from build123d import *

# Parameters (mm, degrees)
PAD_DEPTH = 8


with BuildPart() as part:
    # Sketch → Pad (new body)
    with BuildSketch(Plane.XY):
        with BuildLine():
            ThreePointArc((-29.53026, 52.229912), (0, -60), (29.53026, 52.229912))
            Line((29.53026, 122.229912), (29.53026, 52.229912))
            Line((23.53026, 122.229912), (29.53026, 122.229912))
            Line((23.53026, 122.229912), (23.53026, 82.229912))
            Line((23.53026, 82.229912), (-29.53026, 52.229912))
        make_face()
    extrude(amount=PAD_DEPTH)


solid = part.part
Here's how the part is built. I have some questions about the finished solid (model axes, mm). A direction names the side the tool comes from. Give positions to 0.01 mm unless a question says otherwise; leave off trailing zeros. Order: outer loops, then holes, each group sorted by start corner. A loop starts at its lowest first (then second) coordinate and runs counter-clockwise, first axis right, second up. Notation, with made-up numbers: M -27.75,75.5 L -1.75,75.5 A29 ccw -1.75,108.5 Z; hole C 71.5,25.25 d5. An arc over 180 degrees is marked long. Answer as a JSON object with one key per item and string values. Group by question number.
1) Please list where these lines run through material, in increasing order: L1, parallel to X at y = 84.5, z = 5.5; L2, parallel to Y at x = 12.5, z = 2; L3, parallel to Y at x = -46, z = 5.5. Write a range as [from, to].
2) Suppose I cut it at B-B, the plane x = 44.5. Write out the boundary of the cut face in (y, z), plus the area to 3 significant figures.
3) Suppose I cut it at A-A, the plane y = 93. Write out the boundary of the cut face in (x, z), plus the area to 3 significant figures.
4) On a 3-axis mill with a long thin cutter (end or side, diameter ignored), from which of +Z, -Z, +X, -X, +Y, -Y can I reach the whole of each face in a straight line? I mean faces 1 (the flat face through (29.53, 88, 4)), 2 (the flat face through (23.53, 103, 4)), 3 (the flat face through (-1, 12, 8)). Say none if no direction works.
5) I'm going to push flat-ended pins straight in: pin 1 Ø1.5 at (y, z) = (-7.5, 3) entering from +X; pin 2 Ø4 at (x, z) = (39.5, 6.5) entering from +Y; pin 3 Ø1 at (x, z) = (-19.5, 4.5) entering from -Y. Where does each tip first touch, or does it pass through?
Results found:
{
 "1": {"L1": "[23.53, 29.53]", "L2": "[-58.68, 75.99]", "L3": "[-38.52, 38.52]"},
 "2": {"outline": "M -40.25,0 L 40.25,0 L 40.25,8 L -40.25,8 Z", "area": "644 mm²"},
 "3": {"outline": "M 23.53,0 L 29.53,0 L 29.53,8 L 23.53,8 Z", "area": "48.0 mm²"},
 "4": {"face 1": "+Z, -Z, +X, +Y", "face 2": "+Z, -Z, -X, +Y", "face 3": "+Z, +X, -X, +Y, -Y"},
 "5": {"pin 1": "x = 59.62", "pin 2": "y = 46.84", "pin 3": "y = -56.91"}
}
